Here's how the part is built. I have some questions about the finished solid (model axes, mm). Give positions to 0.01 mm unless a question says otherwise; leave off trailing zeros. Loops run counter-clockwise (first coordinate to the right, second up) from the corner with the lowest first, then second, coordinate; pieces in that order, holes last.
Q1. If we section it at A-A (x = 20): Please give me the cut outline in (y, z).
Q2. I need wall thicknesses on line 1 (Z direction, x = 12, y = 38); line 2 (Y direction, x = 21, z = 1.5); line 3 (Y direction, x = 20, z = 1.1). Which ranges of each line are inside material? Lowest first, please.
Q3. Will these pins go through, and if not, where does the flat tip stop? P1, Ø1, axis at x = 15.5, z = -1, coming from the +Y side; P2, Ø3.5, axis at x = 37, y = 3, coming from the -Z side; P3, Ø2, axis at x = 32, y = 6.5, coming from the -Z side.
Q4. If we section it at C-C (x = 10): Please give me the cut outline in (y, z).
Q5. If we section it at D-D (x = 3): Please give me the cut outline in (y, z).
Q6. If we section it at B-B (y = 29): Please give me the cut outline in (x, z).
from build123d import *

# Parameters (mm, degrees)
F0_W      = 40
F0_H      = 40
F1_DEPTH  = 3
F2_R      = 18
F3_DEPTH  = 3.001
F4_R      = 2
F5_DEPTH  = 3.001
F7_DEPTH  = 40
F8_R      = 5
F9_R      = 2.5
F10_DEPTH = 38.969286
F11_R     = 3


with BuildPart() as f1:
    # F0 (on Top) → F1 (new body)
    with BuildSketch(Plane.XY):
        with Locations((20, 20)):
            Rectangle(F0_W, F0_H)
    extrude(amount=F1_DEPTH)

    # F2 (on face) → F3 (cut, through all)
    with BuildSketch(Plane.XY.offset(3)):
        with Locations((20, 20)):
            Circle(F2_R)
    extrude(amount=-F3_DEPTH, mode=Mode.SUBTRACT)

    # F4 (on face) → F5 (cut, through all)
    with BuildSketch(Plane.XY.offset(3)):
        with Locations((3, 37)):
            Circle(F4_R)
        with Locations((3, 3)):
            Circle(F4_R)
        with Locations((37, 37)):
            Circle(F4_R)
        with Locations((37, 3)):
            Circle(F4_R)
    extrude(amount=-F5_DEPTH, mode=Mode.SUBTRACT)

    # F6 (on face) → F7 (join)
    with BuildSketch(Plane.YZ.offset(40)):
        Polygon((43.002259, 2.997741), (40, 3), (43, 0), (50.608861, -7.608861), (53.608861, -7.608861), align=None)
        Polygon((43, 0), (40, 3), (40, 0), align=None)
        Polygon((52.108244, -9.109478), (53.608861, -7.608861), (50.608861, -7.608861), align=None)
    extrude(amount=-F7_DEPTH)

    # F8
    f8_edges = [f1.edges().sort_by_distance(p)[0] for p in [
        (20, 43.002259, 2.997741),
    ]]
    fillet(f8_edges, radius=F8_R)

    # F9 (on face) → F10 (cut, through all)
    with BuildSketch(Plane(origin=(0, 23, 23), x_dir=(1, 0, 0), z_dir=(0, 0.707107, 0.707107))):
        with Locations((30, 36.787466)):
            Circle(F9_R)
        with Locations((10, 36.787466)):
            Circle(F9_R)
    extrude(amount=-F10_DEPTH, mode=Mode.SUBTRACT)

    # F11
    f11_edges = [f1.edges().sort_by_distance(p)[0] for p in [
        (20, 43, 0),
    ]]
    fillet(f11_edges, radius=F11_R)


solid = f1.part
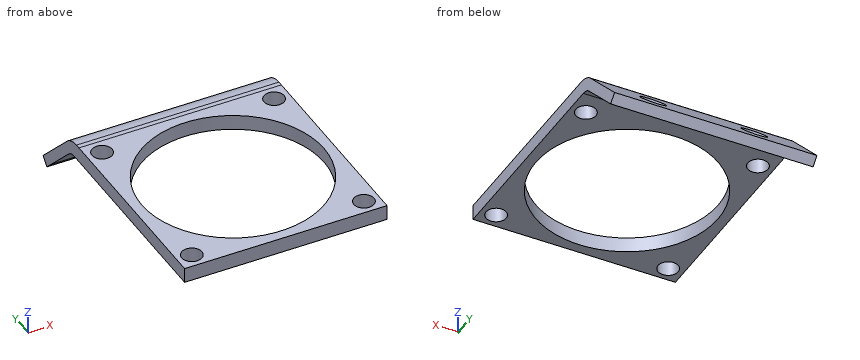
Check sheet entries:
1. outline: (0, 0) - (2, 0) - (2, 3) - (0, 3) - close; (38, 0) - (41.76, 0) arc R3 cw to (43.88, -0.88) - (50.61, -7.61) - (52.11, -9.11) - (53.61, -7.61) - (44.47, 1.53) arc R5 ccw to (40.93, 3) - (40, 3) - (38, 3) - close
2. line 1: z = 0 to 3
2. line 2: y = 0 to 2.03, 37.97 to 44.5
2. line 3: y = 0 to 2, 38 to 44.9
3. P1: stops at y = 47.5
3. P2: passes through
3. P3: stops at z = 0
4. outline: (0, 0) - (5.03, 0) - (5.03, 3) - (0, 3) - close; (34.97, 0) - (41.76, 0) arc R3 cw to (43.88, -0.88) - (45.74, -2.74) - (47.24, -1.24) - (44.47, 1.53) arc R5 ccw to (40.93, 3) - (40, 3) - (34.97, 3) - close; (49.28, -6.28) - (50.61, -7.61) - (52.11, -9.11) - (53.61, -7.61) - (50.78, -4.78) - close
5. outline: (0, 0) - (1, 0) - (1, 3) - (0, 3) - close; (5, 0) - (14.08, 0) - (14.08, 3) - (5, 3) - close; (25.92, 0) - (35, 0) - (35, 3) - (25.92, 3) - close; (39, 0) - (41.76, 0) arc R3 cw to (43.88, -0.88) - (50.61, -7.61) - (52.11, -9.11) - (53.61, -7.61) - (44.47, 1.53) arc R5 ccw to (40.93, 3) - (40, 3) - (39, 3) - close
6. outline: (0, 0) - (4.41, 0) - (4.41, 3) - (0, 3) - close; (35.59, 0) - (40, 0) - (40, 3) - (35.59, 3) - close
